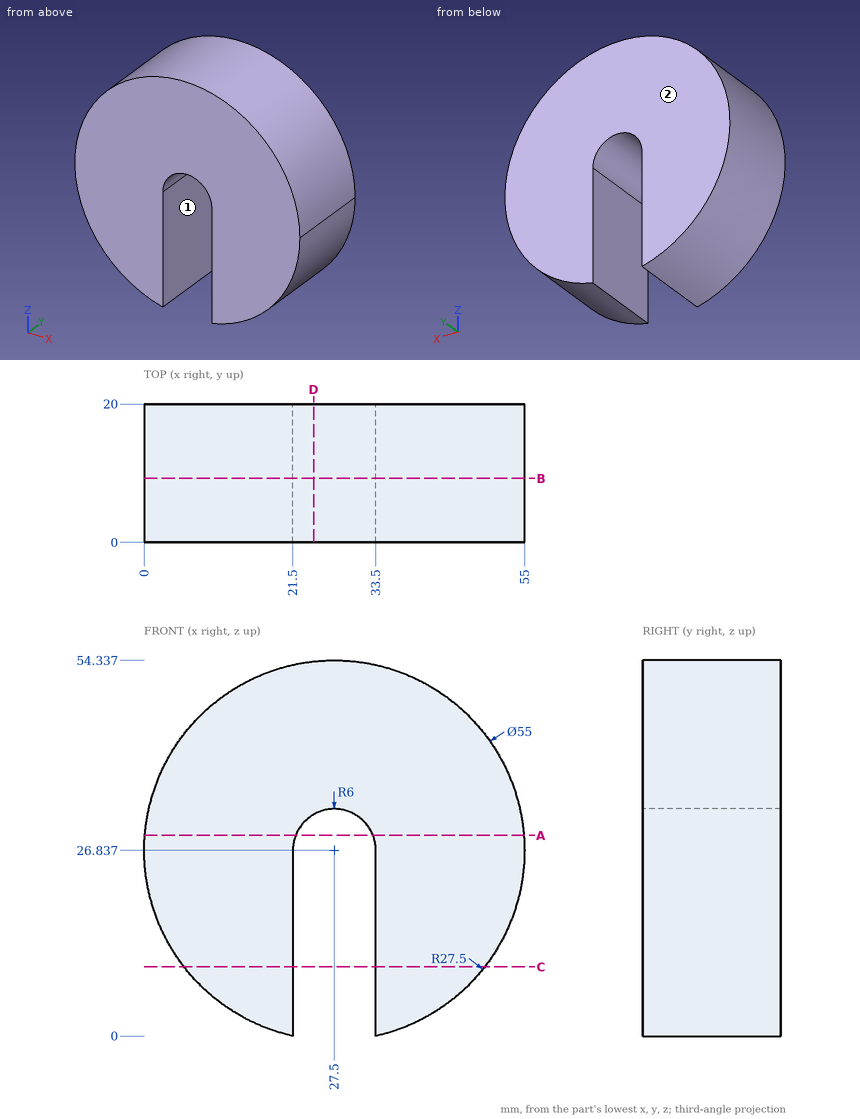
Check sheet for the drawn part. Datum: minimum x, y, z corner. Units: mm. A direction names the side the tool comes from. Round coordinates to 2 decimals unless told otherwise and drop trailing zeros. Loops run counter-clockwise (first coordinate to the right, second up) from the corner with the lowest first, then second, coordinate; pieces in that order, holes last. Notation, with made-up numbers: (84.5, 13) -> (94.5, 13) arc R15 cw to (94.5, 40) -> close; hole circle Ø1 at (6, 64). An arc over 180 degrees is marked (long way). Put each result on its own line as item: value. Start each with the question number.
1. Section check B-B (y = 9.25). Enter the section's corners in (x, z), plus the area to 3 significant figures.
2. Section check D-D (x = 24.5). Enter the section's corners in (y, z), plus the area to 3 significant figures.
3. Access from +Z, -Z, +X, -X, +Y, -Y to the whole of each face (thin tool, end or side, straight path). Record for the marked faces 1 and 2.
4. Section check A-A (z = 29). Enter the section's corners in (x, y) (1 decimal), plus the area to 3 significant figures.
5. Section check C-C (z = 10). Enter the section's corners in (x, y), plus the area to 3 significant figures.
6. Gauge pin test, flat ends, axial feed: pin 1 (2 mm diameter, centred on x = 30, y = 5.5, fed in from +Z); pin 2 (10 mm diameter, centred on y = 16.5, z = 22, fed in from +X); pin 3 (4 mm diameter, centred on x = 7, y = 18, fed in from -Z); pin 4 (10 mm diameter, centred on y = 8, z = 8.5, fed in from -X). Record the tip position at first contact, or that the pin passes through.
7. Scan lines: probe 1 along X at (y, z) = (5.5, 27); probe 2 along X at (y, z) = (13.5, 31) (1 decimal); probe 3 along Z at (x, y) = (16.5, 6.75) (1 decimal). Record each from-to range of solid material in increasing order.
Findings:
1. outline: (21.5, 0) -> (21.5, 26.84) arc R6 cw to (33.5, 26.84) -> (33.5, 0) arc R27.5 ccw (long way) to start
1. area: 1,990 mm^2
2. outline: (0, 32.03) -> (20, 32.03) -> (20, 54.17) -> (0, 54.17) -> close
2. area: 443 mm^2
3. face 1: -Z, +Y, -Y
3. face 2: +Z, -Z, +X, -X, +Y
4. outline: (0.1, 0) -> (21.9, 0) -> (21.9, 20) -> (0.1, 20) -> close; (33.1, 0) -> (54.9, 0) -> (54.9, 20) -> (33.1, 20) -> close
4. area: 873 mm^2
5. outline: (5.76, 0) -> (21.5, 0) -> (21.5, 20) -> (5.76, 20) -> close; (33.5, 0) -> (49.24, 0) -> (49.24, 20) -> (33.5, 20) -> close
5. area: 630 mm^2
6. pin 1: stops at z = 54.3
6. pin 2: stops at x = 55
6. pin 3: stops at z = 6.49
6. pin 4: stops at x = 3.45
7. probe 1: x = 0 to 21.5, 33.5 to 55
7. probe 2: x = 0.3 to 23.2, 31.8 to 54.7
7. probe 3: z = 1.6 to 52
